Autodesk Inventor part; units mm, degrees
ref_plane "YZ Plane" through (0, 0, 0) normal (1, 0, 0) x (0, 1, 0)
ref_plane "XZ Plane" through (0, 0, 0) normal (0, 1, 0) x (-1, 0, 0)
ref_plane "XY Plane" through (0, 0, 0) normal (0, 0, 1) x (1, 0, 0)
sketch "Sketch1" plane through (0, 0, 0) normal (1, 0, 0) x (0, 1, 0)
  circle A0 centre (0, 0) radius 6.35
  dimension "d0" = 12.7
extrude "Extrusion1" add sketch "Sketch1" along normal blind 9.5
sketch "Sketch2" plane through (9.5, 0, 0) normal (1, 0, 0) x (0, 0, -1)
  circle A0 centre (0, 0) radius 1.5875
  dimension "d3" = 3.175
extrude "Extrusion2" add sketch "Sketch2" along normal blind 12.5
sketch "Sketch3" plane through (0, 0, 0) normal (-1, 0, 0) x (0, 0, 1)
  line L0 (-0.8, 2.3) -> (0.8, 2.3)
  line L1 (0.8, 2.3) -> (0.8, 2)
  line L2 (0.8, 2) -> (-0.8, 2)
  line L3 (-0.8, 2) -> (-0.8, 2.3)
  line L4 (-3.34, -2.78) -> (-1.74, -2.78)
  line L5 (-1.74, -2.78) -> (-1.74, -3.08)
  line L6 (-1.74, -3.08) -> (-3.34, -3.08)
  line L7 (-3.34, -3.08) -> (-3.34, -2.78)
  line L8 (1.74, -2.78) -> (3.34, -2.78)
  line L9 (3.34, -2.78) -> (3.34, -3.08)
  line L10 (3.34, -3.08) -> (1.74, -3.08)
  line L11 (1.74, -3.08) -> (1.74, -2.78)
  point P0 (0, 0)
  dimension "d6" = 1.6
  dimension "d7" = 0.3
  dimension "d8" = 0.3
  dimension "d9" = 1.6
  dimension "d10" = 1.6
  dimension "d11" = 0.3
  dimension "d12" = 0.8
  dimension "d13" = 2
  dimension "d14" = 4.78
  dimension "d15" = 0
  dimension "d16" = 3.48
  dimension "d17" = 1.74
extrude "Extrusion3" add sketch "Sketch3" along normal blind 5
sketch "Sketch4" plane through (9.5, 0, 0) normal (1, 0, 0) x (0, 0, -1)
  circle A0 centre (0, 0) radius 3.175
  dimension "d20" = 6.35
extrude "Extrusion4" add sketch "Sketch4" along normal blind 6.35
properties part number "Potentiometer"
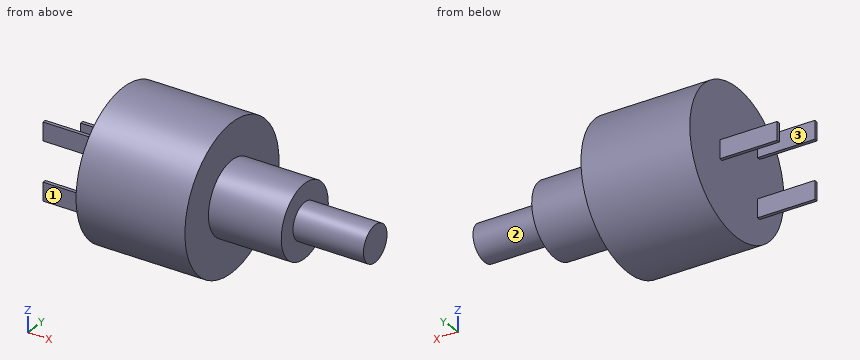
Source: CAD feature listing. Evaluate the final solid. Frame: model axes, mm. Face numbers are marked on the shaded views. A direction names the side the tool comes from. Coordinates: 2 decimals unless noted, no trailing zeros. Order: outer loops, then holes, each group sorted by start corner. A loop starts at its lowest first (then second) coordinate and runs counter-clockwise, first axis right, second up.
Item 1: Cut plane C-C (x = 18). Return loops of the section in (y, z) (1 decimal), plus the area to 3 significant figures.
Output values:
outline: circle Ø3.2 at (0, 0)
area: 7.92 mm2
Item 2: Set-up query: the marked faces 1, 2 and 3. Return all of +Z, -Z, +X, -X, +Y, -Y with unobstructed straight access to the full face (end or side cutting, diameter ignored); none if empty.
Output values:
face 1: +Z, -Z, -X, -Y
face 2: +X
face 3: +Z, -Z, -X, +Y
Item 3: First-contact query: P1, Ø4, axis at y = 0, z = -2.5, coming from the -X side; P2, Ø0.5, axis at x = -3, z = 2.5, coming from the -Y side; P3, Ø5, axis at x = 2, z = 4, coming from the +Y side. Flat tips, straight axial feed; report the tip coordinate or a pass-through.
Output values:
P1: stops at x = 0
P2: stops at y = -3.08
P3: stops at y = 6.17
Item 4: Material intervals for line 1 (X direction, y = -2.75, z = 5.25); line 2 (X direction, y = -2.75, z = 1); line 3 (Z direction, x = 5.25, y = 3.5), sorted ascending.
Output values:
line 1: x = 0 to 9.5
line 2: x = 0 to 15.85
line 3: z = -5.3 to 5.3
Item 5: Cut plane D-D (y = 2.75). Return loops of the section in (x, z).
Output values:
outline: (0, -5.72) - (9.5, -5.72) - (9.5, -1.59) - (15.85, -1.59) - (15.85, 1.59) - (9.5, 1.59) - (9.5, 5.72) - (0, 5.72) - close
